Verification items for the finished model (mm, model axes). A direction names the side the tool comes from. Give positions to 0.01 mm unless a question says otherwise; leave off trailing zeros. Loops run counter-clockwise (first coordinate to the right, second up) from the corner with the lowest first, then second, coordinate; pieces in that order, holes last. Notation, with made-up numbers: (86.25, 48) - (143.25, 48) arc R15 ccw to (143.25, 70) - close; hole circle Ø7 at (87.5, 22.25). An arc over 180 degrees is marked (long way). Use one line per item in the form item = value.
```python
from build123d import *

# Parameters (mm, degrees)
BOSS_EXTRUDE1_DEPTH     = 8
BOSS_EXTRUDE1_2_DEPTH   = 8
SKETCH2_R               = 14
BOSS_EXTRUDE2_DEPTH     = 8
CUT_EXTRUDE1_DEPTH      = 217.781153328
CUT_EXTRUDE1_DEPTH_BACK = 217.781153328
SKETCH3_R               = 2.05
SKETCH3_R_2             = 1.6


with BuildPart() as part:
    # Sketch1 → Boss-Extrude1 (new body)
    with BuildSketch(Plane(origin=(0, 0, 0), x_dir=(1, 0, 0), z_dir=(0, 1, 0))):
        Polygon((12, -9.7155), (64.77, -17.81175), (183.515, -8.31215), (211.582, -3.0226), (215.9, 0), (211.582, 4.5339), (183.515, 6.80085), (64.77, 14.57325), (12, 9.7155), align=None)
    extrude(amount=BOSS_EXTRUDE1_DEPTH)



with BuildPart() as body_2:
    # Sketch1 → Boss-Extrude1 2 (new body)
    with BuildSketch(Plane(origin=(0, 0, 0), x_dir=(1, 0, 0), z_dir=(0, 1, 0))):
        Polygon((-12, -9.7155), (-64.77, -17.81175), (-183.515, -8.31215), (-211.582, -3.0226), (-215.9, 0), (-211.582, 4.5339), (-183.515, 6.80085), (-64.77, 14.57325), (-12, 9.7155), align=None)
    extrude(amount=BOSS_EXTRUDE1_2_DEPTH)


with BuildPart() as part_1:
    add(part.part)

    add(body_2.part)  # Boss-Extrude2 merges body 2
    # Sketch2 → Boss-Extrude2 (add)
    with BuildSketch(Plane(origin=(0, 0, 0), x_dir=(1, 0, 0), z_dir=(0, 1, 0))):
        Circle(SKETCH2_R)
    extrude(amount=BOSS_EXTRUDE2_DEPTH)

    # Sketch3 → Cut-Extrude1 (cut, two sides: drawn at the far end of the back side and taken through both)
    with BuildSketch(Plane(origin=(0, 0, 0), x_dir=(1, 0, 0), z_dir=(0, 1, 0)).offset(-CUT_EXTRUDE1_DEPTH_BACK)):
        with Locations(Location((0, 0, 0), (0, 0, 270))):
            Circle(SKETCH3_R)
        with Locations(Location((6, 0, 0), (0, 0, 270))):
            Circle(SKETCH3_R_2)
        with Locations(Location((-6, 0, 0), (0, 0, 270))):
            Circle(SKETCH3_R_2)
    extrude(amount=CUT_EXTRUDE1_DEPTH + CUT_EXTRUDE1_DEPTH_BACK, mode=Mode.SUBTRACT)


solid = part_1.part
```
1. Tool access check on faces 1 (the flat face through (-3, 0, 1)), 2 (the flat face through (38.754, 3.944, -12.178)), 3 (the flat face through (-38.016, 3.944, 13.707)). Record the directions out of +Z, -Z, +X, -X, +Y, -Y that give a thin tool (end or side, any length) a straight path to the whole face; none if there is none.
Result set:
face_1 = +Z, -Z, +X, -X, -Y
face_2 = -Z, +Y, -Y
face_3 = +Z, +Y, -Y
2. Section check B-B, the plane x = 176.5. Record the cut outline in (y, z).
Result set:
outline = (0, -7.26) - (8, -7.26) - (8, 8.87) - (0, 8.87) - close
3. Draft check along X on faces 4 (the flat face through (38.016, 3.944, 13.707)), 5 (the flat face through (-123.31, 3.94, 13.13)), 6 (the flat face through (-38.754, 3.944, -12.178)), 7 (the flat face through (123.31, 3.94, 13.13)). Enter one of: released by +X, released by -X, zero draft, split by the parting line, or undercut.
Result set:
face_4 = undercut
face_5 = released by -X
face_6 = undercut
face_7 = released by +X
4. Scan lines: probe 1 along X at (y, z) = (3.75, 0); probe 2 along X at (y, z) = (4, 3); probe 3 along Z at (x, y) = (-6, 2.25). Record each from-to range of solid material in increasing order.
Result set:
probe_1 = -215.9 to -7.6, -4.4 to -2.05, 2.05 to 4.4, 7.6 to 215.9
probe_2 = -211.61 to 211.61
probe_3 = -12.65 to -1.6, 1.6 to 12.65
5. Depth check by flat-ended pin: pin 1 Ø3 at (x, z) = (6, 0) entering from +Y; pin 2 Ø3 at (y, z) = (6.5, -2) entering from +X; pin 3 Ø1.5 at (x, y) = (95, 4) entering from +Z. Enter the tip coordinate at first touch or a pass-through.
Result set:
pin_1 = through
pin_2 = 215.42
pin_3 = 15.45
6. Section check A-A, the plane y = 6.5. State how many separate pieces and enclosed holes the cut face has, then the cut area to 3 significant figures.
Result set:
separate_pieces = 1
enclosed_holes = 3
area = 9,590 mm²
